Verification items for the finished model (mm, model axes). A direction names the side the tool comes from. Round coordinates to 2 decimals unless told otherwise and drop trailing zeros. Order: outer loops, then holes, each group sorted by start corner. A loop starts at its lowest first (then second) coordinate and runs counter-clockwise, first axis right, second up. Notation, with made-up numbers: M 15.5,48.5 L 51.5,48.5 A24 ccw 51.5,82.5 Z; hole C 77,-38 d4. An arc over 180 degrees is marked long. Use CSV: the item, a comma, the result in double quotes. Start each with the question number.
Q1. Sectioned sample at A-A (x = 0). Enter the section's corners in (y, z), and give its area (3 significant figures).
Q2. Set-up check for faces 5 (the face through (-11.811, 0, 38)), 6 (the face through (-0.17, -8.9, -6.26)), 7 (the face through (-6.61, 9.79, 37.57)): record each of +Z, -Z, +X, -X, +Y, -Y from which the full face is reachable in a straight line by a thin tool's end or side.
Q3. Sectioned sample at D-D (y = -10.16). Enter the section's corners in (x, z).
Q4. Sectioned sample at B-B (y = 0). Enter the section's corners in (x, z).
Q5. Gauge pin test, flat ends, axial feed: pin 1 Ø5 at (x, z) = (-10, 4.5) entering from +Y; pin 2 Ø3.5 at (x, y) = (0, -10.16) entering from -Z; pin 3 Ø1.5 at (y, z) = (8, 53.5) entering from +X; pin 4 Ø4 at (x, z) = (-9, 40.5) entering from -Y. Record the tip position at first contact, or that the pin passes through.
Q6. Scan lines: line 1 (Y direction, x = 0, z = -8.75); line 2 (Z direction, x = 9.25, y = 2.5); line 3 (X direction, y = 2.25, z = 66.5). Record each from-to range of solid material in increasing order.
Q7. Sectioned sample at C-C (z = 68). Enter the section's corners in (x, y).
Q8. Mould release check, pull along X, two halves, no side actions. Record for faces 1 (the face through (-7.08, 10.62, 21.25)), 2 (the face through (11.811, 0, 38)), 3 (the face through (0, 0, -12.7)), 4 (the face through (0.586, 9.033, -6.261)): +X half, -X half, draft (parallel to the pull), parting line (faces both ways), or undercut.
```python
from build123d import *
from build123d import SkipClean  # not in build123d's __all__

# Parameters (mm, degrees)
F1_R     = 12.7635
F1_R_2   = 1.27
F2_DEPTH = 12.7
F3_DEPTH = 76.2


with BuildPart() as f2:
    # F1 (on Top) → F2 (new body)
    with BuildSketch(Plane.XY):
        Circle(F1_R)
        with Locations((0, -10.16)):
            Circle(F1_R_2, mode=Mode.SUBTRACT)
        with Locations((0, 10.16)):
            Circle(F1_R_2, mode=Mode.SUBTRACT)
    extrude(amount=-F2_DEPTH)

    # F0 (on Top) → F3 (join)
    with BuildSketch(Plane.XY):
        with BuildLine():
            Line((-3.81, 11.1796073724), (-3.81, 12.1815775764))
            ThreePointArc((-3.81, 12.1815775764), (-6.5274436814, 10.9681088268), (-8.89, 9.1583203837))
            Line((-8.89, 9.1583203837), (-8.89, 7.7760929135))
            ThreePointArc((-8.89, 7.7760929135), (-6.5740761836, 9.8123006136), (-3.81, 11.1796073724))
        make_face()
        with BuildLine():
            Line((-11.811, -4.8380999628), (-11.811, 4.8380999628))
            ThreePointArc((-11.811, 4.8380999628), (-12.7635, 0), (-11.811, -4.8380999628))
        make_face()
        with BuildLine():
            ThreePointArc((11.811, -4.8380999628), (12.7635, 0), (11.811, 4.8380999628))
            Line((11.811, 4.8380999628), (11.811, -4.8380999628))
        make_face()
        with BuildLine():
            ThreePointArc((8.89, 9.1583203837), (6.5274436814, 10.9681088268), (3.81, 12.1815775764))
            Line((3.81, 12.1815775764), (3.81, 11.1796073724))
            ThreePointArc((3.81, 11.1796073724), (6.5740761836, 9.8123006136), (8.89, 7.7760929135))
            Line((8.89, 7.7760929135), (8.89, 9.1583203837))
        make_face()
    with SkipClean():  # cleaning this boolean's faces spoils the solid; the shape is the same uncleaned
        extrude(amount=F3_DEPTH)


solid = f2.part
```
Verdict:
1,outline,"M -12.76,-12.7 L -11.43,-12.7 L -11.43,0 L -12.76,0 Z; M -8.89,-12.7 L 8.89,-12.7 L 8.89,0 L -8.89,0 Z; M 11.43,-12.7 L 12.76,-12.7 L 12.76,0 L 11.43,0 Z"
1,area,"260 mm²"
2,face 5,"+Z, +Y, -Y"
2,face 6,"+Z, -Z"
2,face 7,"+Z, -Y"
3,outline,"M -7.73,-12.7 L -1.27,-12.7 L -1.27,0 L -7.73,0 Z; M 1.27,-12.7 L 7.73,-12.7 L 7.73,0 L 1.27,0 Z"
4,outline,"M -12.76,-12.7 L 12.76,-12.7 L 12.76,76.2 L 11.81,76.2 L 11.81,0 L -11.81,0 L -11.81,76.2 L -12.76,76.2 Z"
5,pin 1,"stops at y = 10.33"
5,pin 2,"stops at z = -12.7"
5,pin 3,"stops at x = 8.89"
5,pin 4,"stops at y = 7.78"
6,line 1,"y = -12.76 to -11.43, -8.89 to 8.89, 11.43 to 12.76"
6,line 2,"z = -12.7 to 0"
6,line 3,"x = -12.56 to -11.81, 11.81 to 12.56"
7,outline,"M -11.81,-4.84 L -11.81,4.84 A12.76 ccw Z; M -8.89,7.78 A11.81 cw -3.81,11.18 L -3.81,12.18 A12.76 ccw -8.89,9.16 Z; M 3.81,11.18 A11.81 cw 8.89,7.78 L 8.89,9.16 A12.76 ccw 3.81,12.18 Z; M 11.81,-4.84 A12.76 ccw 11.81,4.84 Z"
8,face 1,"parting line"
8,face 2,"undercut"
8,face 3,"draft"
8,face 4,"undercut"
